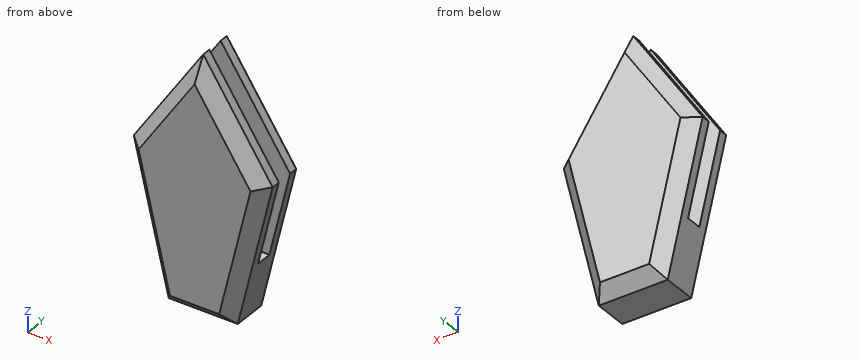
from build123d import *

# Parameters (mm, degrees)
F1_DEPTH = 4.7
F2_W     = 1.3
F2_H     = 20
F3_DEPTH = 10
F4_SIZE  = 1


with BuildPart() as f1:
    # F0 (on Front) → F1 (new body)
    with BuildSketch(Plane.XZ):
        Polygon((-5.535933, 11.672128), (-2.75, 0), (2.75, 0), (5.535933, 11.672128), (0, 20), align=None)
    extrude(amount=F1_DEPTH)

    # F2 (on Right) → F3 (cut, symmetric)
    with BuildSketch(Plane.YZ):
        with Locations((-2.35, 14.75)):
            Rectangle(F2_W, F2_H)
    extrude(amount=F3_DEPTH, both=True, mode=Mode.SUBTRACT)

    # F4
    f4_edges = [f1.edges().sort_by_distance(p)[0] for p in [
        (-4.142966, -4.7, 5.836064),
        (0, -4.7, 0),
        (4.142966, -4.7, 5.836064),
        (2.767966, -4.7, 15.836064),
        (-2.767966, -4.7, 15.836064),
        (-4.142966, 0, 5.836064),
        (0, 0, 0),
        (4.142966, 0, 5.836064),
        (2.767966, 0, 15.836064),
        (-2.767966, 0, 15.836064),
    ]]
    chamfer(f4_edges, length=F4_SIZE)


solid = f1.part
Here's how the part is built. I have some questions about the finished solid (model axes, mm). Coordinates: 2 decimals unless noted, no trailing zeros. Order: outer loops, then holes, each group sorted by start corner. A loop starts at its lowest first (then second) coordinate and runs counter-clockwise, first axis right, second up. Notation, with made-up numbers: M 55,13.25 L 65,13.25 A18 ccw 65,32.25 Z; hole C 84.5,50.25 d4. An arc over 180 degrees is marked long. Answer as CSV lines item,"result".
Item 1: If I drill on line 1 (Y direction, x = 0, z = 13); line 2 (Y direction, x = -4, z = 7.5); line 3 (Z direction, x = 0.5, y = -1.75), over which ranges is the centre line in solid material (lowest first)?
Results found:
line 1,"-4.7 to -3, -1.7 to 0"
line 2,"-4.23 to -3, -1.7 to -0.47"
line 3,"0 to 4.75"
Item 2: Imagine slicing it at A-A on z = 14. Write out the boundary of the cut face in (x, y), plus the area to 3 significant figures.
Results found:
outline,"M -3.99,-3.7 L -2.79,-4.7 L 2.79,-4.7 L 3.99,-3.7 L 3.99,-3 L -3.99,-3 Z; M -3.99,-1.7 L 3.99,-1.7 L 3.99,-1 L 2.79,0 L -2.79,0 L -3.99,-1 Z"
area,"24.7 mm2"
Item 3: Imagine slicing it at D-D on z = 3.75. Write out the boundary of the cut face in (x, y).
Results found:
outline,"M -3.65,-3.7 L -2.62,-4.7 L 2.62,-4.7 L 3.65,-3.7 L 3.65,-1 L 2.62,0 L -2.62,0 L -3.65,-1 Z"
Item 4: Imagine slicing it at C-C on y = -2.15. Write out the boundary of the cut face in (x, z).
Results found:
outline,"M -3.88,4.75 L -2.75,0 L 2.75,0 L 3.88,4.75 Z"
Item 5: Imagine slicing it at B-B on x = -3.5. Write out the boundary of the cut face in (y, z).
Results found:
outline,"M -4.7,7.45 L -3.7,3.14 L -1,3.14 L 0,7.45 L 0,12.93 L -1,14.73 L -1.7,14.73 L -1.7,4.75 L -3,4.75 L -3,14.73 L -3.7,14.73 L -4.7,12.93 Z"
Item 6: For pin 1 (1.5 mm diameter, centred on y = -2, z = 16, fed in from +X); pin 2 (0.6 mm diameter, centred on x = 1.5, y = -2.5, fed in from +Z), each with a flat end and sliding along its axis, tell me the tip position at first contact or that it passes through.
Results found:
pin 1,"x = 3.12"
pin 2,"z = 4.75"
